from build123d import *

# Parameters (mm, degrees)
F1_DEPTH = 25.25
F2_R     = 25
F3_DEPTH = 49.9
F4_R     = 26
F5_DEPTH = 9
F6_R     = 7.45
F7_DEPTH = 10


with BuildPart() as f1:
    # F0 (on Front) → F1 (new body)
    with BuildSketch(Plane.XZ):
        with BuildLine():
            Line((0, 0), (26.1, 0))
            ThreePointArc((26.1, 0), (0, 26.1), (-26.1, 0))
            Line((-26.1, 0), (0, 0))
        make_face()
        with BuildLine():
            ThreePointArc((-26.1, 0), (0, -26.1), (26.1, 0))
            Line((26.1, 0), (0, 0))
            Line((0, 0), (-26.1, 0))
        make_face()
    extrude(amount=-F1_DEPTH)

    # F2 (on face) → F3 (join)
    with BuildSketch(Plane(origin=(0, 25.25, 0), x_dir=(-1, 0, 0), z_dir=(0, 1, 0))):
        Circle(F2_R)
    extrude(amount=F3_DEPTH)

    # F4 (on face) → F5 (join)
    with BuildSketch(Plane(origin=(0, 75.15, 0), x_dir=(-1, 0, 0), z_dir=(0, 1, 0))):
        Circle(F4_R)
    extrude(amount=F5_DEPTH)

    # F6 (on face) → F7 (join)
    with BuildSketch(Plane(origin=(0, 84.15, 0), x_dir=(-1, 0, 0), z_dir=(0, 1, 0))):
        Circle(F6_R)
    extrude(amount=F7_DEPTH)


solid = f1.part
Here's how the part is built. I have some questions about the finished solid (model axes, mm). A direction names the side the tool comes from. Round coordinates to 2 decimals unless told otherwise and drop trailing zeros. Write each loop counter-clockwise with the first axis right and the second up, starting at its lowest first coordinate (ties: lowest second). Pieces come first, ordered by that corner, then holes.
1. If we mould it in two halves opening along Y, with no side actions, what happens to faces 3 (the flat face through (0, 94.15, 0)), 4 (the cylindrical face through (-23.846, 49.851, 7.509)), 5 (the flat face through (14, 75.15, 21)), 6 (the cylindrical face through (5.66, 12.45, 25.48))? For each: released by +Y, released by -Y, zero draft, split by the parting line, or undercut.
2. I need wall thicknesses on L1, parallel to Y at x = 15.5, z = 12.5; L2, parallel to Y at x = -20, z = 16; L3, parallel to X at y = 42, z = 0.5 (3 decimals). Which ranges of each line are inside material? Lowest first, please.
3. Suppose I cut it at B-B (x = 0). List the corners of the cut face in (y, z) for me.
4. Suppose I cut it at D-D (z = 13.5). List the corners of the cut face in (x, y) for me.
5. Suppose I cut it at C-C (y = 66). List the corners of the cut face in (x, z) for me.
6. For faces 1 (the flat face through (0, 0, 0)), 2 (the flat face through (-5.4, 84.15, -5.4)), which set-ups out of +Z, -Z, +X, -X, +Y, -Y let a thin tool reach every point of the face, with its end or its side?
7. Suppose I cut it at A-A (z = 0). List the corners of the cut face in (x, y) for me, and give its area (3 significant figures).
8. Will these pins go through, and if not, where does the flat tip stop? pin 1 Ø4 at (y, z) = (66, -3) entering from +X; pin 2 Ø1 at (x, y) = (-16.5, 44) entering from +Z; pin 3 Ø12 at (y, z) = (57, -4.5) entering from -X.
Answer sheet:
1. face 3: released by +Y
1. face 4: undercut
1. face 5: undercut
1. face 6: zero draft
2. L1: y = 0 to 84.15
2. L2: y = 0 to 25.25, 75.15 to 84.15
2. L3: x = -24.995 to 24.995
3. outline: (0, -26.1) - (25.25, -26.1) - (25.25, -25) - (75.15, -25) - (75.15, -26) - (84.15, -26) - (84.15, -7.45) - (94.15, -7.45) - (94.15, 7.45) - (84.15, 7.45) - (84.15, 26) - (75.15, 26) - (75.15, 25) - (25.25, 25) - (25.25, 26.1) - (0, 26.1) - close
4. outline: (-22.34, 0) - (22.34, 0) - (22.34, 25.25) - (21.04, 25.25) - (21.04, 75.15) - (22.22, 75.15) - (22.22, 84.15) - (-22.22, 84.15) - (-22.22, 75.15) - (-21.04, 75.15) - (-21.04, 25.25) - (-22.34, 25.25) - close
5. outline: circle Ø50 at (0, 0)
6. face 1: +Z, -Z, +X, -X, -Y
6. face 2: +Y
7. outline: (-26.1, 0) - (26.1, 0) - (26.1, 25.25) - (25, 25.25) - (25, 75.15) - (26, 75.15) - (26, 84.15) - (7.45, 84.15) - (7.45, 94.15) - (-7.45, 94.15) - (-7.45, 84.15) - (-26, 84.15) - (-26, 75.15) - (-25, 75.15) - (-25, 25.25) - (-26.1, 25.25) - close
7. area: 4,430 mm2
8. pin 1: stops at x = 24.98
8. pin 2: stops at z = 19.21
8. pin 3: stops at x = -25
